Check sheet for the modelled part. Datum: model origin and axes. Units: mm. A direction names the side the tool comes from. Round coordinates to 2 decimals unless told otherwise and drop trailing zeros. Write each loop counter-clockwise with the first axis right and the second up, starting at its lowest first coordinate (ties: lowest second). Pieces come first, ordered by that corner, then holes. Notation, with made-up numbers: (2, 33.25) -> (19, 33.25) arc R4 ccw to (19, 38.25) -> close; hole circle Ø1 at (11, 50). An arc over 180 degrees is marked (long way). One line per item, written item: value.
from build123d import *

# Parameters (mm, degrees)
SKIZZE1_W                       = 20
SKIZZE1_H                       = 20
AUFSATZ_LINEAR_AUSTRAGEN1_DEPTH = 100
SCHNITT_LINEAR_AUSTRAGEN1_DEPTH = 104.923048454
SKETCH1_R                       = 3
EXTRUDE1_DEPTH                  = 104.923048454


with BuildPart() as part:
    # Skizze1 → Aufsatz-Linear austragen1 (new body)
    with BuildSketch(Plane(origin=(0, 0, 0), x_dir=(1, 0, 0), z_dir=(0, 1, 0))):
        with Locations((10, 10)):
            Rectangle(SKIZZE1_W, SKIZZE1_H)
    extrude(amount=AUFSATZ_LINEAR_AUSTRAGEN1_DEPTH)

    # Skizze2 → Schnitt-Linear austragen1 (cut, through all)
    with BuildSketch(Plane(origin=(0, 100, 0), x_dir=(1, 0, 0), z_dir=(0, 1, 0))):
        Polygon((7, 20), (10, 17), (13, 20), align=None)
        Polygon((20, 13), (17, 10), (20, 7), align=None)
        Polygon((0, 7), (0, 13), (3, 10), align=None)
        Polygon((7, 0), (13, 0), (10, 3), align=None)
    extrude(amount=-SCHNITT_LINEAR_AUSTRAGEN1_DEPTH, mode=Mode.SUBTRACT)

    # Sketch1 → Extrude1 (cut, through all)
    with BuildSketch(Plane(origin=(0, 100, 0), x_dir=(1, 0, 0), z_dir=(0, 1, 0))):
        with Locations(Location((10, 10, 0), (0, 0, 270))):
            Circle(SKETCH1_R)
    extrude(amount=-EXTRUDE1_DEPTH, mode=Mode.SUBTRACT)


solid = part.part
Item 1: Sectioned sample at A-A (z = -18.25). Enter the section's corners in (x, y), then the cut area to 3 significant figures.
Result set:
outline: (0, 0) -> (8.75, 0) -> (8.75, 100) -> (0, 100) -> close; (11.25, 0) -> (20, 0) -> (20, 100) -> (11.25, 100) -> close
area: 1,750 mm^2
Item 2: Release check for a two-part mould opening along Z. For faces 5 (the flat face through (3, 49, -20)), 6 (the flat face through (1, 51, -12)), 7 (the flat face through (7.6, 0, -12.4)) record: pulls with the +Z half, pulls with the -Z half, needs draft (parallel to the pull), parting line crosses it, or undercut.
Result set:
face 5: pulls with the -Z half
face 6: undercut
face 7: needs draft
Item 3: Depth check by flat-ended pin: pin 1 (3.5 mm diameter, centred on x = 10, z = -10, fed in from -Y) (3 decimals). Enter the tip coordinate at first touch or a pass-through.
Result set:
pin 1: through
Item 4: Sectioned sample at B-B (y = 78). Enter the section's corners in (x, z).
Result set:
outline: (0, -20) -> (7, -20) -> (10, -17) -> (13, -20) -> (20, -20) -> (20, -13) -> (17, -10) -> (20, -7) -> (20, 0) -> (13, 0) -> (10, -3) -> (7, 0) -> (0, 0) -> (0, -7) -> (3, -10) -> (0, -13) -> close; hole circle Ø6 at (10, -10)
Item 5: Tool access check on faces 1 (the flat face through (9, 51, -2)), 2 (the flat face through (18, 51, -9)), 3 (the flat face through (2, 51, -9)), 4 (the flat face through (11, 51, -18)). Record the directions out of +Z, -Z, +X, -X, +Y, -Y that give a thin tool (end or side, any length) a straight path to the whole face; none if there is none.
Result set:
face 1: +Z, +Y, -Y
face 2: +X, +Y, -Y
face 3: -X, +Y, -Y
face 4: -Z, +Y, -Y
Item 6: Sectioned sample at C-C (z = -8.75). Enter the section's corners in (x, y), then the cut area to 3 significant figures.
Result set:
outline: (1.75, 0) -> (7.27, 0) -> (7.27, 100) -> (1.75, 100) -> close; (12.73, 0) -> (18.25, 0) -> (18.25, 100) -> (12.73, 100) -> close
area: 1,100 mm^2
Item 7: Material ranges on line 1 along X through (y, z) = (74, -10); line 2 along Z through (x, y) = (11.5, 93); line 3 along Z through (x, y) = (1.5, 7), recorded low to high.
Result set:
line 1: 3 to 7, 13 to 17
line 2: -18.5 to -12.6, -7.4 to -1.5
line 3: -20 to -11.5, -8.5 to 0
